Here's how the part is built. I have some questions about the finished solid (model axes, mm). A direction names the side the tool comes from. Give positions to 0.01 mm unless a question says otherwise; leave off trailing zeros. Order: outer loops, then holes, each group sorted by start corner. A loop starts at its lowest first (then second) coordinate and runs counter-clockwise, first axis right, second up. Notation, with made-up numbers: (52.25, -23) -> (80.25, -23) arc R28 cw to (80.25, 13) -> close; hole circle Ø1 at (57, 68.5). An arc over 180 degrees is marked (long way). Write each question's results on one line, items separated by ' | '. Start each with the question number.
Q1. I'm going to push flat-ended pins straight in: pin 1 (4 mm diameter, centred on x = -3, y = 5, fed in from +Z); pin 2 (2 mm diameter, centred on y = 6, z = 0.5, fed in from +X); pin 3 (1.3 mm diameter, centred on y = 8, z = -1, fed in from -X); pin 4 (3.5 mm diameter, centred on x = 1, z = 0, fed in from -Y). Where does each tip first touch, or does it pass through?
Q2. Imagine slicing it at B-B, the plane y = 20. Please give me the cut outline in (x, z), then the cut area to 3 significant figures.
Q3. I need wall thicknesses on line 1 along X through (y, z) = (8, -2); line 2 along Z through (x, y) = (5, 1); line 3 along X through (y, z) = (13.75, -2.75). Which ranges of each line are inside material? Lowest first, please. Write a range as [from, to].
Q4. Imagine slicing it at A-A, the plane x = 0. Please give me the cut outline in (y, z).
Q5. Imagine slicing it at D-D, the plane y = 10.25. Please give me the cut outline in (x, z).
Q6. Imagine slicing it at C-C, the plane z = -0.75. Please give me the cut outline in (x, y), then the cut area to 3 significant figures.
Q7. For faces 1 (the face through (-6.25, 7, 0)), 2 (the face through (0, 7, -2.25)), 3 (the face through (0, 7, 2.25)), which set-ups out of +Z, -Z, +X, -X, +Y, -Y let a thin tool reach every point of the face, with its end or its side?
```python
from build123d import *

# Parameters (mm, degrees)
SKETCH1_W           = 12.5
SKETCH1_H           = 4.5
BOSS_EXTRUDE1_DEPTH = 13.4
BOSS_EXTRUDE2_DEPTH = 3.5


with BuildPart() as part:
    # Sketch1 → Boss-Extrude1 (new body)
    with BuildSketch(Plane(origin=(0, 0, 0), x_dir=(1, 0, 0), z_dir=(0, 1, 0))):
        Rectangle(SKETCH1_W, SKETCH1_H)
    extrude(amount=BOSS_EXTRUDE1_DEPTH)

    # Sketch2 → Boss-Extrude2 (add, symmetric)
    with BuildSketch(Plane.XY):
        with BuildLine():
            Line((-11, 13.4), (11, 13.4))
            ThreePointArc((11, 13.4), (0, 24.4), (-11, 13.4))
        make_face()
    extrude(amount=BOSS_EXTRUDE2_DEPTH, both=True)


solid = part.part
```
Geometry check:
1) pin 1: z = 2.25 | pin 2: x = 6.25 | pin 3: x = -6.25 | pin 4: y = 0
2) outline: (-8.8, -3.5) -> (8.8, -3.5) -> (8.8, 3.5) -> (-8.8, 3.5) -> close | area: 123 mm²
3) line 1: [-6.25, 6.25] | line 2: [-2.25, 2.25] | line 3: [-10.99, 10.99]
4) outline: (0, -2.25) -> (13.4, -2.25) -> (13.4, -3.5) -> (24.4, -3.5) -> (24.4, 3.5) -> (13.4, 3.5) -> (13.4, 2.25) -> (0, 2.25) -> close
5) outline: (-6.25, -2.25) -> (6.25, -2.25) -> (6.25, 2.25) -> (-6.25, 2.25) -> close
6) outline: (-11, 13.4) -> (-6.25, 13.4) -> (-6.25, 0) -> (6.25, 0) -> (6.25, 13.4) -> (11, 13.4) arc R11 ccw to start | area: 358 mm²
7) face 1: +Z, -Z, -X, -Y | face 2: -Z, +X, -X, -Y | face 3: +Z, +X, -X, -Y
